Work out the finished part from the listing and answer in its coordinate system (mm). A direction names the side the tool comes from. Round coordinates to 2 decimals unless told otherwise and drop trailing zeros. Order: outer loops, then holes, each group sorted by start corner. A loop starts at its lowest first (then second) coordinate and runs counter-clockwise, first axis right, second up. Notation, with made-up numbers: (19, 76) - (55, 76) arc R25 ccw to (55, 114) - close; hole circle Ø9 at (4.25, 44.25). An arc over 180 degrees is marked (long way). Answer in a Markdown table with one row per item.
from build123d import *

# Parameters (mm, degrees)
F0_R      = 17.145
F1_DEPTH  = 3.81
F2_R      = 13.716
F2_R_2    = 11.43
F3_DEPTH  = 0.254
F4_DEPTH  = 0.762
F5_R      = 5.715
F6_DEPTH  = 0.762
F8_R      = 1.905
F9_DEPTH  = 25.4
F10_R     = 2.413
F11_DEPTH = 2.032
F14_R     = 3.175
F15_DEPTH = 8.89
F16_R     = 1.905
F17_DEPTH = 8.89
F18_R     = 0.508
F19_R     = 0.508
F20_R     = 13.208
F20_R_2   = 10.668
F21_DEPTH = 0.254
F22_DEPTH = 0.508


# Not quite as in the source:
# - the program builds the solid bodies; features that only make, move or delete a surface that nothing else refers to are left out


with BuildPart() as f1:
    # F0 (on Front) → F1 (new body)
    with BuildSketch(Plane.XZ):
        Circle(F0_R)
    extrude(amount=F1_DEPTH)

    # F2 (on face) → F3 (cut)
    with BuildSketch(Plane.XZ.offset(3.81)):
        Circle(F2_R)
        Circle(F2_R_2, mode=Mode.SUBTRACT)
    extrude(amount=-F3_DEPTH, mode=Mode.SUBTRACT)

    # F4 (cut): a face of the model
    f4_faces = [f1.faces().sort_by_distance(p)[0] for p in [
        (0, -3.81, 0),
    ]]
    extrude(f4_faces, amount=-F4_DEPTH, mode=Mode.SUBTRACT)

    # F5 (on face) → F6 (join)
    with BuildSketch(Plane.XZ.offset(3.048)):
        Circle(F5_R)
    extrude(amount=F6_DEPTH)

    # F8 (on face) → F9 (cut)
    with BuildSketch(Plane.XZ.offset(3.048)):
        with Locations((0, 8.1100180022)):
            Circle(F8_R)
        with Locations((-5.7346487249, 5.7346487249)):
            Circle(F8_R)
        with Locations((-5.7346487249, -5.7346487249)):
            Circle(F8_R)
        with Locations((0, -8.1100180022)):
            Circle(F8_R)
        with Locations((5.7346487249, -5.7346487249)):
            Circle(F8_R)
        with Locations((8.1100180022, 0)):
            Circle(F8_R)
        with Locations((5.7346487249, 5.7346487249)):
            Circle(F8_R)
        with Locations((-8.1100180022, 0)):
            Circle(F8_R)
    extrude(amount=-F9_DEPTH, mode=Mode.SUBTRACT)

    # F10 (on face) → F11 (join)
    with BuildSketch(Plane.XZ.offset(3.81)):
        Circle(F10_R)
    extrude(amount=F11_DEPTH)

    # F14 (on Front) → F15 (join)
    with BuildSketch(Plane.XZ):
        Circle(F14_R)
    extrude(amount=-F15_DEPTH)

    # F16 (on face) → F17 (cut)
    with BuildSketch(Plane(origin=(0, 8.89, 0), x_dir=(-1, 0, 0), z_dir=(0, 1, 0))):
        Circle(F16_R)
    extrude(amount=-F17_DEPTH, mode=Mode.SUBTRACT)

    # F18
    f18_edges = [f1.edges().sort_by_distance(p)[0] for p in [
        (-17.145, -3.81, 0),
    ]]
    fillet(f18_edges, radius=F18_R)

    # F19
    f19_edges = [f1.edges().sort_by_distance(p)[0] for p in [
        (-17.145, 0, 0),
    ]]
    fillet(f19_edges, radius=F19_R)

    # F20 (on face) → F21 (cut)
    with BuildSketch(Plane(origin=(0, 0, 0), x_dir=(-1, 0, 0), z_dir=(0, 1, 0))):
        Circle(F20_R)
        Circle(F20_R_2, mode=Mode.SUBTRACT)
    extrude(amount=-F21_DEPTH, mode=Mode.SUBTRACT)

    # F22 (cut): a face of the model
    f22_faces = [f1.faces().sort_by_distance(p)[0] for p in [
        (10.3662633943, 0, 0),
    ]]
    extrude(f22_faces, amount=-F22_DEPTH, mode=Mode.SUBTRACT)


solid = f1.part
1) Which of the six approach directions +Z, -Z, +X, -X, +Y, -Y give full straight-line access (tool end or side, diameter ignored) to faces 4 (the face through (-5.983, -1.796, 7.623)), 5 (the face through (-1, -0.254, 11)), 6 (the face through (5.45, -3.42, 1.72))?
Filled in:
| item | result |
|---|---|
| face 4 | +Y, -Y |
| face 5 | +Y |
| face 6 | -Y |
2) Find section A-A, the plane x = 0. Give the number of separate pieces and of enclosed holes in the cut face, then the cut area to 3 significant figures.
Filled in:
| item | result |
|---|---|
| separate pieces | 3 |
| enclosed holes | 0 |
| area | 125 mm^2 |
3) The mould has two halves that part along X. Classify faces 1 (the face through (-5.24, -3.048, 2.7)), 2 (the face through (-1.915, -4.812, -1.468)), 3 (the face through (1.2, -3.81, -2.5)): released by +X, released by -X, zero draft, split by the parting line, or undercut.
Filled in:
| item | result |
|---|---|
| face 1 | undercut |
| face 2 | split by the parting line |
| face 3 | zero draft |
4) Find section B-B, the plane y = 3.5. Give the vertices of the cut face in (x, z) (3 decimals).
Filled in:
| item | result |
|---|---|
| outline | circle Ø6.35 at (0, 0); hole circle Ø3.81 at (0, 0) |
5) Each of these flat-tipped pins is pushed along its axis until it touches: pin 1 (8 mm diameter, centred on x = -13, y = 1.5, fed in from +Z); pin 2 (3 mm diameter, centred on y = 7, z = -3, fed in from -X); pin 3 (4 mm diameter, centred on x = -5.5, z = 1.5, fed in from -Y); pin 4 (3.5 mm diameter, centred on x = -8.11, z = 0, fed in from -Y). Where does it stop, or does it pass through?
Filled in:
| item | result |
|---|---|
| pin 1 | stops at z = 14.27 |
| pin 2 | stops at x = -2.8 |
| pin 3 | stops at y = -3.81 |
| pin 4 | passes through |
6) Find the intervals of material crossed by probe 1 along Z at (x, y) = (0, -1.25) (3 decimals); probe 2 along Z at (x, y) = (5.5, -2.5); probe 3 along X at (y, z) = (-1, 5), in increasing order. Write a range as from..to.
Filled in:
| item | result |
|---|---|
| probe 1 | z = -17.145..-10.015, -6.205..6.205, 10.015..17.145 |
| probe 2 | z = -16.24..-7.63, -3.84..3.84, 7.63..16.24 |
| probe 3 | x = -16.4..-7.49, -3.98..3.98, 7.49..16.4 |
